Geometry: final body of the model. Coordinates: model frame, mm. A direction names the side the tool comes from. Give positions to 0.01 mm unless a question says otherwise; leave off trailing zeros. Order: outer loops, then holes, each group sorted by start corner. A loop starts at its lowest first (then second) coordinate and runs counter-clockwise, first axis right, second up. Notation, with made-up numbers: (61, 34) -> (80, 34) arc R21 ccw to (80, 48) -> close; hole circle Ø10 at (41, 86.25). An arc over 180 degrees is marked (long way). One line per item, written item: value. Start each with the question number.
```python
from build123d import *

# Parameters (mm, degrees)
BOSS_EXTRUDE1_DEPTH = 6.6
SKETCH2_5_W         = 76.6
SKETCH2_5_H         = 84.22
CUT_EXTRUDE9_DEPTH  = 1.6
CUT_EXTRUDE10_DEPTH = 3
SKETCH2_R           = 1.55
CUT_EXTRUDE3_DEPTH  = 90.468527235
FILLET1_R           = 5
SKETCH5_R           = 1.525
CUT_EXTRUDE4_DEPTH  = 10
SKETCH5_3_R         = 4.5
CUT_EXTRUDE5_DEPTH  = 1
CUT_EXTRUDE6_DEPTH  = 2.4


with BuildPart() as part:
    # Sketch1 → Boss-Extrude1 (new body)
    with BuildSketch(Plane(origin=(0, 0, 0), x_dir=(1, 0, 0), z_dir=(0, 1, 0))):
        Polygon((-36.907015775, 45.377886591), (-36.907015775, -14.842113409), (-56.907015775, -14.842113409), (-56.907015775, -29.842113409), (-44.307015775, -29.842113409), (45.692984225, -29.842113409), (65.692984225, -29.842113409), (65.692984225, -14.842113409), (45.692984225, -14.842113409), (45.692984225, 45.377886591), (65.692984225, 45.377886591), (65.692984225, 60.377886591), (45.692984225, 60.377886591), (-44.307015775, 60.377886591), (-56.907015775, 60.377886591), (-56.907015775, 45.377886591), align=None)
    extrude(amount=BOSS_EXTRUDE1_DEPTH)

    # Sketch2_5 → Cut-Extrude9 (cut)
    with BuildSketch(Plane(origin=(0, 6.6, 0), x_dir=(1, 0, 0), z_dir=(0, 1, 0))):
        with Locations((4.392984225, 15.267886591)):
            Rectangle(SKETCH2_5_W, SKETCH2_5_H)
    extrude(amount=-CUT_EXTRUDE9_DEPTH, mode=Mode.SUBTRACT)

    # Sketch11 → Cut-Extrude10 (cut)
    with BuildSketch(Plane(origin=(0, 5, 0), x_dir=(1, 0, 0), z_dir=(0, 1, 0))):
        Polygon((-18.907015775, 50.377886591), (-18.907015775, -13.842113409), (-23.907015775, -13.842113409), (-23.907015775, -26.842113409), (-11.907015775, -26.842113409), (-11.907015775, -6.842113409), (11.092984225, -6.842113409), (11.092984225, -23.842113409), (31.092984225, -23.842113409), (31.092984225, -17.842113409), (40.692984225, -17.842113409), (40.692984225, 42.377886591), (28.692984225, 42.377886591), (28.692984225, 50.377886591), align=None)
    extrude(amount=-CUT_EXTRUDE10_DEPTH, mode=Mode.SUBTRACT)

    # Sketch2 → Cut-Extrude3 (cut, through all)
    with BuildSketch(Plane(origin=(0, 6.6, 0), x_dir=(1, 0, 0), z_dir=(0, 1, 0))):
        with Locations(Location((38.682984225, 53.367886591, 0), (0, 0, 270))):
            Circle(SKETCH2_R)
        with Locations(Location((-29.897015775, 53.367886591, 0), (0, 0, 270))):
            Circle(SKETCH2_R)
        with Locations(Location((-29.897015775, -22.832113409, 0), (0, 0, 270))):
            Circle(SKETCH2_R)
        with Locations(Location((38.682984225, -22.832113409, 0), (0, 0, 270))):
            Circle(SKETCH2_R)
    extrude(amount=-CUT_EXTRUDE3_DEPTH, mode=Mode.SUBTRACT)

    # Fillet1
    fillet1_edges = [part.edges().sort_by_distance(p)[0] for p in [
        (65.692984225, 3.3, -60.377886591),
        (65.692984225, 3.3, -45.377886591),
        (45.692984225, 3.3, -45.377886591),
        (45.692984225, 3.3, 14.842113409),
        (65.692984225, 3.3, 14.842113409),
        (65.692984225, 3.3, 29.842113409),
        (-56.907015775, 3.3, 29.842113409),
        (-56.907015775, 3.3, 14.842113409),
        (-36.907015775, 3.3, 14.842113409),
        (-36.907015775, 3.3, -45.377886591),
        (-56.907015775, 3.3, -45.377886591),
        (-56.907015775, 3.3, -60.377886591),
    ]]
    fillet(fillet1_edges, radius=FILLET1_R)

    # Sketch5 → Cut-Extrude4 (cut)
    with BuildSketch(Plane(origin=(0, 6.6, 0), x_dir=(1, 0, 0), z_dir=(0, 1, 0))):
        with Locations(Location((-49.407015775, 52.877886591, 0), (0, 0, 270))):
            Circle(SKETCH5_R)
        with Locations(Location((-49.407015775, -22.342113409, 0), (0, 0, 270))):
            Circle(SKETCH5_R)
        with Locations(Location((58.192984225, -22.342113409, 0), (0, 0, 270))):
            Circle(SKETCH5_R)
        with Locations(Location((58.192984225, 52.877886591, 0), (0, 0, 270))):
            Circle(SKETCH5_R)
    extrude(amount=-CUT_EXTRUDE4_DEPTH, mode=Mode.SUBTRACT)

    # Sketch5_3 → Cut-Extrude5 (cut)
    with BuildSketch(Plane(origin=(0, 6.6, 0), x_dir=(1, 0, 0), z_dir=(0, 1, 0))):
        with Locations(Location((-49.407015775, 52.877886591, 0), (0, 0, 270))):
            Circle(SKETCH5_3_R)
    extrude(amount=-CUT_EXTRUDE5_DEPTH, mode=Mode.SUBTRACT)

    # Sketch6 → Cut-Extrude6 (cut)
    with BuildSketch(Plane.XZ):
        Polygon((-52.610843031, 22.396802624), (-51.056291653, 19.594862223), (-47.852464396, 19.540173008), (-46.203188518, 22.287424193), (-47.757739897, 25.089364595), (-50.961567153, 25.14405381), align=None)
        Polygon((58.333022061, 25.543345891), (55.49065449, 24.064005973), (55.350616655, 20.862773491), (58.05294639, 19.140880927), (60.895313961, 20.620220845), (61.035351796, 23.821453327), align=None)
        Polygon((60.566668821, -50.725417907), (57.515733962, -49.745981088), (55.142049366, -51.898449773), (55.819299629, -55.030355276), (58.870234489, -56.009792094), (61.243919085, -53.85732341), align=None)
        Polygon((-52.611149193, -52.845807944), (-51.036863407, -55.636708205), (-47.832729989, -55.668786852), (-46.202882357, -52.909965238), (-47.777168142, -50.119064978), (-50.98130156, -50.086986331), align=None)
        Polygon((-26.956477298, 21.559033103), (-27.32422665, 24.742154278), (-30.264765127, 26.015234584), (-32.837554252, 24.105193715), (-32.469804899, 20.92207254), (-29.529266422, 19.648992234), align=None)
        Polygon((41.318077345, 21.008988549), (41.579403227, 24.202608562), (38.944310108, 26.025733421), (36.047891106, 24.655238268), (35.786565223, 21.461618256), (38.421658342, 19.638493396), align=None)
        Polygon((41.435867732, -55.007744024), (41.479584174, -51.803748257), (38.726700668, -50.163890825), (35.930100719, -51.728029158), (35.886384277, -54.932024925), (38.639267783, -56.571882358), align=None)
        Polygon((-26.703291591, -53.627936278), (-28.074944048, -50.732065159), (-31.268668231, -50.472015472), (-33.090739958, -53.107836904), (-31.719087502, -56.003708023), (-28.525363318, -56.26375771), align=None)
    extrude(amount=-CUT_EXTRUDE6_DEPTH, mode=Mode.SUBTRACT)


solid = part.part
```
1. Draft query along X for faces 1 (the flat face through (45.693, 3, -15)), 2 (the flat face through (-56.907, 3, 22)), 3 (the flat face through (56.346, 1.183, -50.807)). Return one class per face: pulls with the +X half, pulls with the -X half, needs draft (parallel to the pull), parting line crosses it, or undercut.
2. Cut plane C-C, the plane y = 1. State how many separate pieces and enclosed holes the cut face has, then the cut area to 3 significant figures.
3. Material intervals for L1, parallel to X at y = 4.5, z = 5; L2, parallel to X at y = 6.25, z = -25.5; L3, parallel to Z at x = 27, y = 3, sorted ascending. Write a range as [from, to].
4. Cut plane B-B, the plane x = -6.5. Return loops of the section in (y, z), then the cut area to 3 significant figures.
5. Cut plane A-A, the plane z = -25.5. Return loops of the section in (x, y).
6. Pin query (flat end, axial travel): P1, Ø5, axis at x = 10, z = -3.5, coming from the -Y side; P2, Ø1.8, axis at y = 6, z = -32.5, coming from the -X side; P3, Ø3.5, axis at x = 38.68, z = -53.37, coming from the +Y side; P4, Ø3, axis at x = -15.5, z = -11.5, coming from the +Y side. Return the tip coordinate at first contact, or that it passes through.
7. Access query for faces 4 (the flat face through (-28.77, 1.18, 25.37)), 5 (the flat face through (-47, 3, -45.378)), 6 (the flat face through (40.693, 4, -12)). Directions: +Z, -Z, +X, -X, +Y, -Y. A direction counts if a zero-diameter tool reaches every point of the face in a straight line with its end or side. Return the directions, or none.
Answers follow:
1. face 1: pulls with the +X half
1. face 2: pulls with the -X half
1. face 3: undercut
2. separate pieces: 1
2. enclosed holes: 8
2. area: 8,420 mm²
3. L1: x = [-36.91, -18.91], [40.69, 45.69]
3. L2: x = [-36.91, -33.91], [42.69, 45.69]
3. L3: z = [-60.38, -50.38], [23.84, 29.84]
4. outline: (0, -60.38) -> (6.6, -60.38) -> (6.6, -57.38) -> (5, -57.38) -> (5, -50.38) -> (2, -50.38) -> (2, 6.84) -> (5, 6.84) -> (5, 26.84) -> (6.6, 26.84) -> (6.6, 29.84) -> (0, 29.84) -> close
4. area: 289 mm²
5. outline: (-36.91, 0) -> (45.69, 0) -> (45.69, 6.6) -> (42.69, 6.6) -> (42.69, 5) -> (40.69, 5) -> (40.69, 2) -> (-18.91, 2) -> (-18.91, 5) -> (-33.91, 5) -> (-33.91, 6.6) -> (-36.91, 6.6) -> close
6. P1: stops at y = 0
6. P2: stops at x = -36.91
6. P3: stops at y = 5
6. P4: stops at y = 2
7. face 4: -Y
7. face 5: -X, +Y, -Y
7. face 6: +Y
